The listing builds one solid part. Answer for the finished solid, in the listing's coordinates (mm). Give positions to 0.01 mm unless a question says otherwise; leave off trailing zeros. Write each loop counter-clockwise with the first axis right and the second up, starting at its lowest first coordinate (ties: lowest second). Pieces come first, ordered by that corner, then holes.
```python
from build123d import *

# Parameters (mm, degrees)
F0_W     = 215.9
F0_H     = 107.95
F1_DEPTH = 2.54
F2_R     = 15.0114
F2_W     = 21.336
F2_H     = 37.592
F2_R_2   = 6.35
F3_DEPTH = 25.4
F4_W     = 15.875
F4_H     = 25.4
F4_W_2   = 15.588598
F4_H_2   = 39.783249
F5_DEPTH = 25.4
F6_W     = 9.954944
F6_H     = 31.75
F7_DEPTH = 25.4


with BuildPart() as f1:
    # F0 (on Top) → F1 (new body)
    with BuildSketch(Plane.XY):
        with Locations((107.95, -53.975)):
            Rectangle(F0_W, F0_H)
    extrude(amount=F1_DEPTH)

    # F2 (on face) → F3 (cut)
    with BuildSketch(Plane.XY):
        with Locations((39.7979, -26.005359)):
            Circle(F2_R)
        with Locations((39.7979, -77.462117)):
            Rectangle(F2_W, F2_H)
        with Locations((85.7719, -77.462117)):
            Rectangle(F2_W, F2_H)
        with Locations((131.7459, -77.462117)):
            Rectangle(F2_W, F2_H)
        with Locations((177.7199, -77.462117)):
            Rectangle(F2_W, F2_H)
        with Locations((131.603076, -25.982544)):
            Circle(F2_R_2)
    extrude(amount=F3_DEPTH, mode=Mode.SUBTRACT)

    # F4 (on face) → F5 (cut)
    with BuildSketch(Plane.XY.offset(2.54)):
        with Locations((9.5377, -25.4)):
            Rectangle(F4_W, F4_H)
        with BuildLine():
            Line((17.4752, -87.323474), (9.954944, -87.323474))
            ThreePointArc((9.954944, -87.323474), (1.603036, -95.462154), (10.377918, -103.142904))
            Line((10.377918, -103.142904), (17.4752, -103.142904))
            Line((17.4752, -103.142904), (17.4752, -87.323474))
        make_face()
        with Locations((206.3623, -25.4)):
            Rectangle(F4_W, F4_H)
        with Locations((206.219099, -83.631156)):
            Rectangle(F4_W_2, F4_H_2)
    extrude(amount=-F5_DEPTH, mode=Mode.SUBTRACT)

    # F6 (on face) → F7 (cut)
    with BuildSketch(Plane.XY.offset(2.54)):
        with Locations((4.977472, -67.070287)):
            Rectangle(F6_W, F6_H)
    extrude(amount=-F7_DEPTH, mode=Mode.SUBTRACT)


solid = f1.part
```
Item 1: A cutting plane is placed at A-A, the plane y = -36. Give the vertices of the cut face in (x, z).
Conclusion:
outline: (0, 0) - (1.6, 0) - (1.6, 2.54) - (0, 2.54) - close; (17.48, 0) - (28.6, 0) - (28.6, 2.54) - (17.48, 2.54) - close; (51, 0) - (198.42, 0) - (198.42, 2.54) - (51, 2.54) - close; (214.3, 0) - (215.9, 0) - (215.9, 2.54) - (214.3, 2.54) - close
Item 2: Determine the mould class of faces 1 (the face through (24.8, -25.35, 1.25)), 2 (the face through (1.6, -95.3, 1.3)), 3 (the face through (106, -53, 0)) for opening direction X: pulls with the +X half, pulls with the -X half, needs draft (parallel to the pull), parting line crosses it, or undercut.
Conclusion:
face 1: undercut
face 2: undercut
face 3: needs draft
Item 3: A cutting plane is placed at C-C, the plane x = 34. Give the vertices of the cut face in (y, z).
Conclusion:
outline: (-107.95, 0) - (-96.26, 0) - (-96.26, 2.54) - (-107.95, 2.54) - close; (-58.67, 0) - (-39.85, 0) - (-39.85, 2.54) - (-58.67, 2.54) - close; (-12.16, 0) - (0, 0) - (0, 2.54) - (-12.16, 2.54) - close
Item 4: A cutting plane is placed at B-B, the plane x = 85. Give the vertices of the cut face in (y, z).
Conclusion:
outline: (-107.95, 0) - (-96.26, 0) - (-96.26, 2.54) - (-107.95, 2.54) - close; (-58.67, 0) - (0, 0) - (0, 2.54) - (-58.67, 2.54) - close
Item 5: A cutting plane is placed at D-D, the plane z = 1.05. Count the separate pieces of the cut face and the enclosed holes in it, plus the area to 3 significant figures.
Conclusion:
separate pieces: 1
enclosed holes: 10
area: 17,300 mm2
Item 6: Each of these flat-tipped pins is pushed along its axis until it touches: P1, Ø1.3, axis at y = -27.5, z = 1, coming from the -X side; P2, Ø12.5, axis at x = 9.54, y = -95.25, coming from the -Z side. Where does it stop, or does it pass through?
Conclusion:
P1: stops at x = 0
P2: passes through
Item 7: Consider probe 1 along X at (y, z) = (-71.5, 2.3); probe 2 along Y at (x, z) = (188, 1.1); probe 3 along X at (y, z) = (-61, 1.2). Determine where each line is inside the solid, lowest interval first.
Conclusion:
probe 1: x = 9.95 to 29.13, 50.47 to 75.1, 96.44 to 121.08, 142.41 to 167.05, 188.39 to 198.42, 214.01 to 215.9
probe 2: y = -107.95 to -96.26, -58.67 to 0
probe 3: x = 9.95 to 29.13, 50.47 to 75.1, 96.44 to 121.08, 142.41 to 167.05, 188.39 to 215.9
